Design review of the part built by this model. Coordinates are the model's own, in mm. Face numbers are marked on the shaded views. A direction names the side the tool comes from. Coordinates: 2 decimals unless noted, no trailing zeros. Write each loop counter-clockwise with the first axis right and the second up, starting at its lowest first coordinate (ties: lowest second). Pieces come first, ordered by that corner, then holes. Notation, with made-up numbers: M -3,12 L 4,12 A25 ccw 4,46 Z; hole C -7.75,-15 d10. An arc over 180 degrees is marked long. Write item = value, one per line.
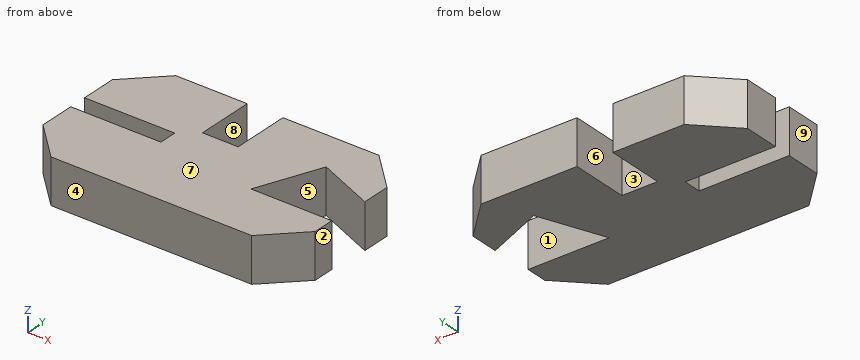
```python
from build123d import *

# Parameters (mm, degrees)
F1_DEPTH = 25
F2_DEPTH = 25


with BuildPart() as f1:
    # F0 (on Top) → F1 (new body)
    with BuildSketch(Plane.XY):
        Polygon((-80.011122, -47.696578), (-60, -67.7077), (52.4, -67.7077), (72.411122, -47.696578), (72.411122, -35.696578), (27.111122, -35.696578), (41.533476, 0), (73.800592, -13.696578), (73.800592, 2.303422), (53.78947, 22.314544), (0, 22.314544), (0, -9.985456), (-20, -9.985456), (-20, 22.314544), (-60, 22.314544), (-80.011122, 2.303422), (-80.011122, -17.696578), (-29.511122, -17.696578), (-29.511122, -27.696578), (-80.011122, -27.696578), align=None)
    extrude(amount=F1_DEPTH)

    # F0 (on Top) → F2 (join)
    with BuildSketch(Plane.XY):
        Polygon((-80.011122, -47.696578), (-60, -67.7077), (52.4, -67.7077), (72.411122, -47.696578), (72.411122, -35.696578), (27.111122, -35.696578), (41.533476, 0), (73.800592, -13.696578), (73.800592, 2.303422), (53.78947, 22.314544), (0, 22.314544), (0, -9.985456), (-20, -9.985456), (-20, 22.314544), (-60, 22.314544), (-80.011122, 2.303422), (-80.011122, -17.696578), (-29.511122, -17.696578), (-29.511122, -27.696578), (-80.011122, -27.696578), align=None)
    extrude(amount=F2_DEPTH)


solid = f1.part
```
Q1. Machinability: for the marked faces 1, 2, 3, 4 and 5, which of the approach directions +Z, -Z, +X, -X, +Y, -Y give a long, thin tool a straight path to every point of the face, cutting with its end or side? Answer none if there is none.
Check result:
face_1 = +Z, -Z, +X
face_2 = +Z, -Z, +X, -Y
face_3 = +Z, -Z, +Y
face_4 = +Z, -Z, +X, -X, -Y
face_5 = +Z, -Z
Q2. For P1, Ø3.5, axis at y = -41.5, z = 15, coming from the +X side; P2, Ø8, axis at x = 58, z = 22.5, coming from the -Y side; P3, Ø5, axis at x = -11, z = 5, coming from the +Y side, all flat-tipped, find the tip position at first contact; note any pin that passes through.
Check result:
P1 = 72.41
P2 = -66.11
P3 = -9.99
Q3. Consider section C-C, the plane z = 12. State the section outline as (x, y) points, and give its area (3 significant figures).
Check result:
outline = M -80.01,-47.7 L -60,-67.71 L 52.4,-67.71 L 72.41,-47.7 L 72.41,-35.7 L 27.11,-35.7 L 41.53,0 L 73.8,-13.7 L 73.8,2.3 L 53.79,22.31 L 0,22.31 L 0,-9.99 L -20,-9.99 L -20,22.31 L -60,22.31 L -80.01,2.3 L -80.01,-17.7 L -29.51,-17.7 L -29.51,-27.7 L -80.01,-27.7 Z
area = 10,700 mm²
Q4. Consider section A-A, the plane x = -49.5. State the section outline as (y, z) points.
Check result:
outline = M -67.71,0 L -27.7,0 L -27.7,25 L -67.71,25 Z; M -17.7,0 L 22.31,0 L 22.31,25 L -17.7,25 Z
Q5. Consider section B-B, the plane y = -3. State the section outline as (x, z) points.
Check result:
outline = M -80.01,0 L -20,0 L -20,25 L -80.01,25 Z; M 0,0 L 40.32,0 L 40.32,25 L 0,25 Z; M 48.6,0 L 73.8,0 L 73.8,25 L 48.6,25 Z
Q6. The part is to be moulded in two halves that separate along X. For the marked faces 6, 7, 8 and 9, say which applies: +X half, -X half, draft (parallel to the pull), parting line (faces both ways), or undercut.
Check result:
face_6 = undercut
face_7 = draft
face_8 = undercut
face_9 = -X half
Q7. Wall thickness on line 1 (X direction, y = -4, z = 22.75); line 2 (Y direction, x = -39.5, z = 16.75); line 3 (Y direction, x = 36, z = 6.5): over which ranges is each line inside the solid? List them lowest first.
Check result:
line_1 = -80.01 to -20, 0 to 39.92, 50.96 to 73.8
line_2 = -67.71 to -27.7, -17.7 to 22.31
line_3 = -67.71 to -35.7, -13.7 to 22.31
Q8. Consider section D-D, the plane y = 13. State the section outline as (x, z) points, and give its area (3 significant figures).
Check result:
outline = M -69.31,0 L -20,0 L -20,25 L -69.31,25 Z; M 0,0 L 63.1,0 L 63.1,25 L 0,25 Z
area = 2,810 mm²
